Read the model definition and answer for the solid it produces. Units are mm, in the model's axes. Face numbers are marked on the shaded views. A direction names the side the tool comes from. Round coordinates to 2 decimals unless told otherwise and drop trailing zeros. Write each loop counter-clockwise with the first axis right and the second up, starting at its lowest first coordinate (ties: lowest second). Pieces come first, ordered by that corner, then holes. Notation, with made-up numbers: (-38.75, 14.25) -> (4.25, 14.25) arc R28 cw to (4.25, 52.25) -> close; hole circle Ø5 at (33, -21.75). An arc over 180 degrees is marked (long way). Return JSON: item names as keys, results as strings.
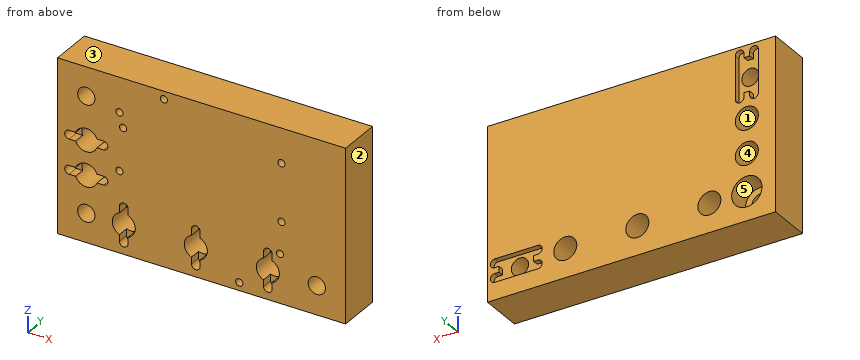
from build123d import *

# Parameters (mm, degrees)
SKETCH1_W             = 100
SKETCH1_H             = 60
BOSS_EXTRUDE1_DEPTH   = 15
CUT_EXTRUDE1_REACH    = 17
SKETCH4_R             = 3
SKETCH5_R             = 5.25
CUT_EXTRUDE2_DEPTH    = 7.7
CUT_EXTRUDE3_REACH    = 17
SKETCH6_R             = 4
CUT_EXTRUDE4_DEPTH    = 4
CUT_EXTRUDE5_REACH    = 17
SKETCH8_R             = 3
CUT_EXTRUDE6_DEPTH    = 2
M3_TAPPED_HOLE1_D     = 2.5
M3_TAPPED_HOLE1_DEPTH = 10
M3_TAPPED_HOLE1_TIP   = 0.751075774


with BuildPart() as part:
    # Sketch1 → Boss-Extrude1 (new body)
    with BuildSketch(Plane(origin=(0, 0, 0), x_dir=(1, 0, 0), z_dir=(0, 1, 0))):
        Rectangle(SKETCH1_W, SKETCH1_H)
    extrude(amount=BOSS_EXTRUDE1_DEPTH)

    # Sketch4 → Cut-Extrude1 (cut, up to next)
    with BuildSketch(Plane(origin=(0, 15, 0), x_dir=(1, 0, 0), z_dir=(0, 1, 0)), mode=Mode.PRIVATE) as cut_extrude1_sk1:
        with Locations((-40, 20)):
            Circle(SKETCH4_R)
    cut_extrude1_tool1 = extrude(cut_extrude1_sk1.sketch, amount=-CUT_EXTRUDE1_REACH, mode=Mode.PRIVATE) & part.part
    add(cut_extrude1_tool1.solids().sort_by_distance((-40, 15, -20))[0], mode=Mode.SUBTRACT)

    # Sketch5 → Cut-Extrude2 (cut)
    with BuildSketch(Plane(origin=(0, 15, 0), x_dir=(1, 0, 0), z_dir=(0, 1, 0))):
        with Locations((-40, 20)):
            Circle(SKETCH5_R)
    extrude(amount=-CUT_EXTRUDE2_DEPTH, mode=Mode.SUBTRACT)

    # Sketch6 → Cut-Extrude3 (cut, up to next)
    with BuildSketch(Plane(origin=(0, 15, 0), x_dir=(1, 0, 0), z_dir=(0, 1, 0)), mode=Mode.PRIVATE) as cut_extrude3_sk1:
        with Locations((-40, 7)):
            Circle(SKETCH6_R)
    cut_extrude3_tool1 = extrude(cut_extrude3_sk1.sketch, amount=-CUT_EXTRUDE3_REACH, mode=Mode.PRIVATE) & part.part
    add(cut_extrude3_tool1.solids().sort_by_distance((-40, 15, -7))[0], mode=Mode.SUBTRACT)
    # Sketch6 → Cut-Extrude3 (cut, up to next)
    with BuildSketch(Plane(origin=(0, 15, 0), x_dir=(1, 0, 0), z_dir=(0, 1, 0)), mode=Mode.PRIVATE) as cut_extrude3_sk2:
        with Locations((-40, -5)):
            Circle(SKETCH6_R)
    cut_extrude3_tool2 = extrude(cut_extrude3_sk2.sketch, amount=-CUT_EXTRUDE3_REACH, mode=Mode.PRIVATE) & part.part
    add(cut_extrude3_tool2.solids().sort_by_distance((-40, 15, 5))[0], mode=Mode.SUBTRACT)
    # Sketch6 → Cut-Extrude3 (cut, up to next)
    with BuildSketch(Plane(origin=(0, 15, 0), x_dir=(1, 0, 0), z_dir=(0, 1, 0)), mode=Mode.PRIVATE) as cut_extrude3_sk3:
        with Locations((-27, 20)):
            Circle(SKETCH6_R)
    cut_extrude3_tool3 = extrude(cut_extrude3_sk3.sketch, amount=-CUT_EXTRUDE3_REACH, mode=Mode.PRIVATE) & part.part
    add(cut_extrude3_tool3.solids().sort_by_distance((-27, 15, -20))[0], mode=Mode.SUBTRACT)
    # Sketch6 → Cut-Extrude3 (cut, up to next)
    with BuildSketch(Plane(origin=(0, 15, 0), x_dir=(1, 0, 0), z_dir=(0, 1, 0)), mode=Mode.PRIVATE) as cut_extrude3_sk4:
        with Locations((-2, 20)):
            Circle(SKETCH6_R)
    cut_extrude3_tool4 = extrude(cut_extrude3_sk4.sketch, amount=-CUT_EXTRUDE3_REACH, mode=Mode.PRIVATE) & part.part
    add(cut_extrude3_tool4.solids().sort_by_distance((-2, 15, -20))[0], mode=Mode.SUBTRACT)
    # Sketch6 → Cut-Extrude3 (cut, up to next)
    with BuildSketch(Plane(origin=(0, 15, 0), x_dir=(1, 0, 0), z_dir=(0, 1, 0)), mode=Mode.PRIVATE) as cut_extrude3_sk5:
        with Locations((23, 20)):
            Circle(SKETCH6_R)
    cut_extrude3_tool5 = extrude(cut_extrude3_sk5.sketch, amount=-CUT_EXTRUDE3_REACH, mode=Mode.PRIVATE) & part.part
    add(cut_extrude3_tool5.solids().sort_by_distance((23, 15, -20))[0], mode=Mode.SUBTRACT)

    # Sketch7 → Cut-Extrude4 (cut)
    with BuildSketch(Plane.XZ):
        with BuildLine():
            Line((-46, 6.5), (-34, 6.5))
            ThreePointArc((-34, 6.5), (-32.5, 5), (-34, 3.5))
            Line((-34, 3.5), (-46, 3.5))
            ThreePointArc((-46, 3.5), (-47.5, 5), (-46, 6.5))
        make_face()
        with BuildLine():
            Line((-46, -5.5), (-34, -5.5))
            ThreePointArc((-34, -5.5), (-32.5, -7), (-34, -8.5))
            Line((-34, -8.5), (-46, -8.5))
            ThreePointArc((-46, -8.5), (-47.5, -7), (-46, -5.5))
        make_face()
        with BuildLine():
            Line((-28.5, -26), (-28.5, -14))
            ThreePointArc((-28.5, -14), (-27, -12.5), (-25.5, -14))
            Line((-25.5, -14), (-25.5, -26))
            ThreePointArc((-25.5, -26), (-27, -27.5), (-28.5, -26))
        make_face()
        with BuildLine():
            Line((-3.5, -26), (-3.5, -14))
            ThreePointArc((-3.5, -14), (-2, -12.5), (-0.5, -14))
            Line((-0.5, -14), (-0.5, -26))
            ThreePointArc((-0.5, -26), (-2, -27.5), (-3.5, -26))
        make_face()
        with BuildLine():
            Line((21.5, -26), (21.5, -14))
            ThreePointArc((21.5, -14), (23, -12.5), (24.5, -14))
            Line((24.5, -14), (24.5, -26))
            ThreePointArc((24.5, -26), (23, -27.5), (21.5, -26))
        make_face()
    extrude(amount=-CUT_EXTRUDE4_DEPTH, mode=Mode.SUBTRACT)

    # Sketch8 → Cut-Extrude5 (cut, up to next)
    with BuildSketch(Plane(origin=(0, 15, 0), x_dir=(1, 0, 0), z_dir=(0, 1, 0)), mode=Mode.PRIVATE) as cut_extrude5_sk1:
        with Locations((40, 20)):
            Circle(SKETCH8_R)
    cut_extrude5_tool1 = extrude(cut_extrude5_sk1.sketch, amount=-CUT_EXTRUDE5_REACH, mode=Mode.PRIVATE) & part.part
    add(cut_extrude5_tool1.solids().sort_by_distance((40, 15, -20))[0], mode=Mode.SUBTRACT)
    # Sketch8 → Cut-Extrude5 (cut, up to next)
    with BuildSketch(Plane(origin=(0, 15, 0), x_dir=(1, 0, 0), z_dir=(0, 1, 0)), mode=Mode.PRIVATE) as cut_extrude5_sk2:
        with Locations((-40, -20)):
            Circle(SKETCH8_R)
    cut_extrude5_tool2 = extrude(cut_extrude5_sk2.sketch, amount=-CUT_EXTRUDE5_REACH, mode=Mode.PRIVATE) & part.part
    add(cut_extrude5_tool2.solids().sort_by_distance((-40, 15, 20))[0], mode=Mode.SUBTRACT)

    # Sketch9 → Cut-Extrude6 (cut)
    with BuildSketch(Plane(origin=(0, 15, 0), x_dir=(1, 0, 0), z_dir=(0, 1, 0))):
        with BuildLine():
            Line((-41, -26), (-42.5, -26))
            Line((-42.5, -26), (-42.5, -21.658312395))
            ThreePointArc((-42.5, -21.658312395), (-43, -20), (-42.5, -18.341687605))
            Line((-42.5, -18.341687605), (-42.5, -14))
            Line((-42.5, -14), (-41, -14))
            Line((-41, -14), (-41, -12.5))
            ThreePointArc((-41, -12.5), (-42.5, -11), (-44, -12.5))
            Line((-44, -12.5), (-44, -27.5))
            ThreePointArc((-44, -27.5), (-42.5, -29), (-41, -27.5))
            Line((-41, -27.5), (-41, -26))
        make_face()
        with BuildLine():
            Line((-41, -14), (-41, -17.171572875))
            ThreePointArc((-41, -17.171572875), (-40, -17), (-39, -17.171572875))
            Line((-39, -17.171572875), (-39, -14))
            Line((-39, -14), (-41, -14))
        make_face()
        with BuildLine():
            Line((-42.5, -21.658312395), (-42.5, -26))
            Line((-42.5, -26), (-41, -26))
            Line((-41, -26), (-41, -22.828427125))
            ThreePointArc((-41, -22.828427125), (-41.84520788, -22.365419176), (-42.5, -21.658312395))
        make_face()
        with BuildLine():
            Line((-41, -22.828427125), (-41, -26))
            Line((-41, -26), (-39, -26))
            Line((-39, -26), (-39, -22.828427125))
            ThreePointArc((-39, -22.828427125), (-40, -23), (-41, -22.828427125))
        make_face()
        with BuildLine():
            Line((-39, -22.828427125), (-39, -26))
            Line((-39, -26), (-37.5, -26))
            Line((-37.5, -26), (-37.5, -21.658312395))
            ThreePointArc((-37.5, -21.658312395), (-38.15479212, -22.365419176), (-39, -22.828427125))
        make_face()
        with BuildLine():
            Line((-37.5, -26), (-39, -26))
            Line((-39, -26), (-39, -27.5))
            ThreePointArc((-39, -27.5), (-37.5, -29), (-36, -27.5))
            Line((-36, -27.5), (-36, -12.5))
            ThreePointArc((-36, -12.5), (-37.5, -11), (-39, -12.5))
            Line((-39, -12.5), (-39, -14))
            Line((-39, -14), (-37.5, -14))
            Line((-37.5, -14), (-37.5, -18.341687605))
            ThreePointArc((-37.5, -18.341687605), (-37.127718677, -19.133974596), (-37, -20))
            ThreePointArc((-37, -20), (-37.127718677, -20.866025404), (-37.5, -21.658312395))
            Line((-37.5, -21.658312395), (-37.5, -26))
        make_face()
        with BuildLine():
            Line((-39, -14), (-39, -17.171572875))
            ThreePointArc((-39, -17.171572875), (-38.15479212, -17.634580824), (-37.5, -18.341687605))
            Line((-37.5, -18.341687605), (-37.5, -14))
            Line((-37.5, -14), (-39, -14))
        make_face()
        with BuildLine():
            Line((-42.5, -14), (-42.5, -18.341687605))
            ThreePointArc((-42.5, -18.341687605), (-41.84520788, -17.634580824), (-41, -17.171572875))
            Line((-41, -17.171572875), (-41, -14))
            Line((-41, -14), (-42.5, -14))
        make_face()
        with BuildLine():
            Line((34, 19), (34, 17.5))
            Line((34, 17.5), (38.341687605, 17.5))
            ThreePointArc((38.341687605, 17.5), (37.634580824, 18.15479212), (37.171572875, 19))
            Line((37.171572875, 19), (34, 19))
        make_face()
        with BuildLine():
            ThreePointArc((42.828427125, 19), (42.365419176, 18.15479212), (41.658312395, 17.5))
            Line((41.658312395, 17.5), (46, 17.5))
            Line((46, 17.5), (46, 19))
            Line((46, 19), (42.828427125, 19))
        make_face()
        with BuildLine():
            Line((38.341687605, 17.5), (34, 17.5))
            Line((34, 17.5), (34, 19))
            Line((34, 19), (32.5, 19))
            ThreePointArc((32.5, 19), (31, 17.5), (32.5, 16))
            Line((32.5, 16), (47.5, 16))
            ThreePointArc((47.5, 16), (49, 17.5), (47.5, 19))
            Line((47.5, 19), (46, 19))
            Line((46, 19), (46, 17.5))
            Line((46, 17.5), (41.658312395, 17.5))
            ThreePointArc((41.658312395, 17.5), (40, 17), (38.341687605, 17.5))
        make_face()
        with BuildLine():
            ThreePointArc((41.658312395, 22.5), (42.365419176, 21.84520788), (42.828427125, 21))
            Line((42.828427125, 21), (46, 21))
            Line((46, 21), (46, 22.5))
            Line((46, 22.5), (41.658312395, 22.5))
        make_face()
        with BuildLine():
            ThreePointArc((43, 20), (42.956795679, 19.492694064), (42.828427125, 19))
            Line((42.828427125, 19), (46, 19))
            Line((46, 19), (46, 21))
            Line((46, 21), (42.828427125, 21))
            ThreePointArc((42.828427125, 21), (42.956795679, 20.507305936), (43, 20))
        make_face()
        with BuildLine():
            Line((34, 21), (34, 19))
            Line((34, 19), (37.171572875, 19))
            ThreePointArc((37.171572875, 19), (37, 20), (37.171572875, 21))
            Line((37.171572875, 21), (34, 21))
        make_face()
        with BuildLine():
            Line((34, 22.5), (34, 21))
            Line((34, 21), (37.171572875, 21))
            ThreePointArc((37.171572875, 21), (37.634580824, 21.84520788), (38.341687605, 22.5))
            Line((38.341687605, 22.5), (34, 22.5))
        make_face()
        with BuildLine():
            Line((32.5, 21), (34, 21))
            Line((34, 21), (34, 22.5))
            Line((34, 22.5), (38.341687605, 22.5))
            ThreePointArc((38.341687605, 22.5), (40, 23), (41.658312395, 22.5))
            Line((41.658312395, 22.5), (46, 22.5))
            Line((46, 22.5), (46, 21))
            Line((46, 21), (47.5, 21))
            ThreePointArc((47.5, 21), (49, 22.5), (47.5, 24))
            Line((47.5, 24), (32.5, 24))
            ThreePointArc((32.5, 24), (31, 22.5), (32.5, 21))
        make_face()
    extrude(amount=-CUT_EXTRUDE6_DEPTH, mode=Mode.SUBTRACT)

    # M3 Tapped Hole1
    with Locations(Plane(origin=(0, 0, 0), x_dir=(-1, 0, 0), z_dir=(0, -1, 0))):
        with Locations((28.5, -18), (27.223611076, -13.081475452), (28.5, 2), (-27.742358719, -18), (-27.742358719, 2), (-27.223611076, 13.081475452), (-13.081475452, 27.223611076), (13.081475452, -27.223611076)):
            Hole(M3_TAPPED_HOLE1_D / 2, depth=M3_TAPPED_HOLE1_DEPTH)
            with Locations((0, 0, -(M3_TAPPED_HOLE1_DEPTH + M3_TAPPED_HOLE1_TIP / 2))):  # 118° drill point
                Cone(0, M3_TAPPED_HOLE1_D / 2, M3_TAPPED_HOLE1_TIP, mode=Mode.SUBTRACT)


solid = part.part
Item 1: For a pull along X with two mould halves and no side action, classify the marked faces 1, 2 and 3 as released by +X, released by -X, zero draft, split by the parting line, or undercut.
Worked answers:
{"face 1": "undercut", "face 2": "released by +X", "face 3": "zero draft"}
Item 2: Section C-C (x = 40) is taken. Give the vertices of the cut face in (y, z).
Worked answers:
{"outline": "(0, -30) -> (15, -30) -> (15, -24) -> (13, -24) -> (13, -23) -> (0, -23) -> close; (0, -17) -> (13, -17) -> (13, -16) -> (15, -16) -> (15, 30) -> (0, 30) -> close"}
Item 3: Section B-B (x = -40) is taken. Give the vertices of the cut face in (y, z), then the cut area to 3 significant figures.
Worked answers:
{"outline": "(0, -30) -> (15, -30) -> (15, -25.25) -> (7.3, -25.25) -> (7.3, -23) -> (0, -23) -> close; (0, -17) -> (7.3, -17) -> (7.3, -14.75) -> (15, -14.75) -> (15, -11) -> (0, -11) -> close; (0, -3) -> (15, -3) -> (15, 1) -> (0, 1) -> close; (0, 9) -> (15, 9) -> (15, 14) -> (13, 14) -> (13, 17) -> (0, 17) -> close; (0, 23) -> (13, 23) -> (13, 26) -> (15, 26) -> (15, 30) -> (0, 30) -> close", "area": "433 mm2"}
Item 4: A tool of negligible diameter and unlimited length cuts with its end or side. For the marked faces 4 and 5, from which of +Z, -Z, +X, -X, +Y, -Y can it reach the whole face along a straight path? Write none if from no direction.
Worked answers:
{"face 4": "+Y, -Y", "face 5": "+Y"}
Item 5: Section D-D (y = 2) is taken. State how many separate pieces and enclosed holes the cut face has, then the cut area to 3 significant figures.
Worked answers:
{"separate pieces": "1", "enclosed holes": "16", "area": "5,530 mm2"}
Item 6: A flat-ended cylindrical pin translates along its axis: pin 1 (2 mm diameter, centred on x = 27.74, z = 18, fed in from -Y). Find the tip coordinate at first contact, or state that the pin passes through.
Worked answers:
{"pin 1": "stops at y = 10.15"}
Item 7: Section A-A (x = -2) is taken. Give the vertices of the cut face in (y, z).
Worked answers:
{"outline": "(0, -30) -> (15, -30) -> (15, -24) -> (4, -24) -> (4, -27.5) -> (0, -27.5) -> close; (0, -12.5) -> (4, -12.5) -> (4, -16) -> (15, -16) -> (15, 30) -> (0, 30) -> close"}
Item 8: Straight lines are drawn through the part: L1, parallel to X at y = 6, z = -20; L2, parallel to Z at x = -40, y = 6.75; L3, parallel to X at y = 11.5, z = -8.5. For each, find the intervals that lie inside material, in ascending order. Write a range as [from, to].
Worked answers:
{"L1": "x = [-50, -43], [-37, -31], [-23, -6], [2, 19], [27, 37], [43, 50]", "L2": "z = [-30, -23], [-17, -11], [-3, 1], [9, 17], [23, 30]", "L3": "x = [-50, -43.71], [-36.29, 50]"}
